Here's how the part is built. I have some questions about the finished solid (model axes, mm). Face numbers are marked on the shaded views. A direction names the side the tool comes from. Coordinates: 2 decimals unless noted, no trailing zeros. Write each loop counter-clockwise with the first axis right and the second up, starting at its lowest first coordinate (ties: lowest second). Pieces come first, ordered by that corner, then holes. Notation, with made-up numbers: (77, 46) -> (86, 46) arc R32 ccw to (86, 74) -> close; hole circle Ø2 at (51, 81.5). An arc over 180 degrees is marked (long way). Put each result on its own line as item: value. Start each with the question number.
Item 1: I want a section at C-C, the plane z = 35. List the corners of the cut face in (x, y) for me, then the cut area to 3 significant figures.
Item 2: I want a section at A-A, the plane x = 17.5. List the corners of the cut face in (y, z) for me.
Item 3: I want a section at D-D, the plane y = -9. List the corners of the cut face in (x, z) for me, then the cut area to 3 significant figures.
Item 4: On a 3-axis mill with a long thin cutter (end or side, diameter ignored), from which of +Z, -Z, +X, -X, +Y, -Y can I reach the whole of each face in a straight line? I mean the marked faces 1 and 2. Say none if no direction works.
Item 5: I need wall thicknesses on line 1 (Y direction, x = 24, z = 35.5); line 2 (Z direction, x = 28, y = -20.5); line 3 (X direction, y = -26, z = 31). Which ranges of each line are inside material? Lowest first, please. Write a range as [from, to].
Item 6: I want a section at B-B, the plane y = -18.5. List the corners of the cut face in (x, z) for me.
Item 7: If we mould it in two halves opening along Z, with no side actions, what happens to the marked faces 3, 4 and 5? For each: released by +Z, released by -Z, zero draft, split by the parting line, or undercut.
Item 8: For pin 1 (1.5 mm diameter, centred on y = -20, z = 9.5, fed in from -X); pin 2 (13.5 mm diameter, centred on y = -15.5, z = 17, fed in from -X), each with a flat end and sliding along its axis, tell me the tip position at first contact or that it passes through.
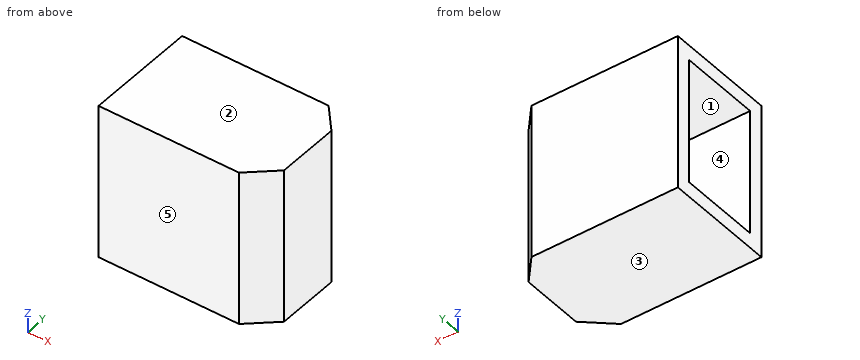
from build123d import *

# Parameters (mm, degrees)
CLOSING_LIP_PROFILE_DEPTH = 52
SHELL_1_T                 = -5


with BuildPart() as part:
    # 草图1 → Closing_lip_profile (new body)
    with BuildSketch(Plane.XY):
        Polygon((-0.915165953, 0), (48, 0), (55, -8), (55, -29), (46, -37), (-0.915165953, -37), align=None)
    extrude(amount=CLOSING_LIP_PROFILE_DEPTH)

    # 抽壳1
    shell_1_openings = [part.faces().sort_by_distance(p)[0] for p in [
        (-0.915165953, -18.5, 26),
    ]]
    offset(amount=SHELL_1_T, openings=shell_1_openings, kind=Kind.INTERSECTION)


solid = part.part
Calculated:
1. outline: (-0.92, -37) -> (46, -37) -> (55, -29) -> (55, -8) -> (48, 0) -> (-0.92, 0) -> (-0.92, -5) -> (45.73, -5) -> (50, -9.88) -> (50, -26.75) -> (44.1, -32) -> (-0.92, -32) -> close
1. area: 656 mm2
2. outline: (-37, 0) -> (0, 0) -> (0, 52) -> (-37, 52) -> close; hole (-32, 5) -> (-5, 5) -> (-5, 47) -> (-32, 47) -> close
3. outline: (-0.92, 0) -> (55, 0) -> (55, 52) -> (-0.92, 52) -> (-0.92, 47) -> (49.23, 47) -> (49.23, 5) -> (-0.92, 5) -> close
3. area: 801 mm2
4. face 1: -X
4. face 2: +Z, +X, -X, +Y, -Y
5. line 1: y = [-37, -32], [-5, 0]
5. line 2: z = [0, 5], [47, 52]
5. line 3: x = [50, 55]
6. outline: (-0.92, 0) -> (55, 0) -> (55, 52) -> (-0.92, 52) -> (-0.92, 47) -> (50, 47) -> (50, 5) -> (-0.92, 5) -> close
7. face 3: released by -Z
7. face 4: undercut
7. face 5: zero draft
8. pin 1: stops at x = 50
8. pin 2: stops at x = 49.01
